The model under review builds one solid part; all positions refer to its coordinate system, in mm. Face numbers are marked on the shaded views. Coordinates: 2 decimals unless noted, no trailing zeros. Write each loop counter-clockwise with the first axis right and the second up, starting at its lowest first coordinate (ties: lowest second). Pieces come first, ordered by that corner, then holes.
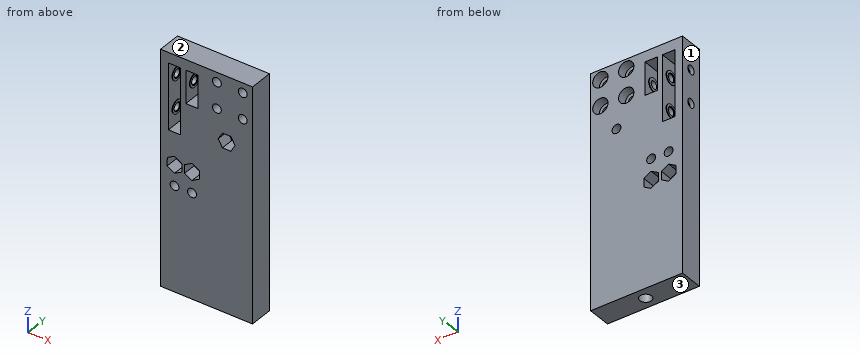
Autodesk Inventor part; units mm, degrees
ref_plane "YZ Plane" through (0, 0, 0) normal (1, 0, 0) x (0, 1, 0)
ref_plane "XZ Plane" through (0, 0, 0) normal (0, 1, 0) x (-1, 0, 0)
ref_plane "XY Plane" through (0, 0, 0) normal (0, 0, 1) x (1, 0, 0)
sketch "Sketch1" plane through (0, 0, 0) normal (0, 1, 0) x (-1, 0, 0)
  line L0 (0, 0) -> (35.5, 0)
  line L1 (35.5, 0) -> (35.5, -90)
  line L2 (35.5, -90) -> (0, -90)
  line L3 (0, -90) -> (0, 0)
  dimension "d0" = 35.5
  dimension "d1" = 90
extrude "Extrusion1" add sketch "Sketch1" along normal blind 9
sketch "Sketch3" plane through (0, 0, 0) normal (0, -1, 0) x (1, 0, 0)
  circle A0 centre (-10, -25) radius 3.25 construction
  line L0 (0, 0) -> (-35.5, 0)
  line L1 (-35.5, 0) -> (-35.5, -90)
  line L2 (-11.6286, -27.8125) -> (-13.25, -24.9958)
  line L3 (-13.25, -24.9958) -> (-11.6214, -22.1833)
  line L4 (-11.6214, -22.1833) -> (-8.3714, -22.1875)
  line L5 (-8.3714, -22.1875) -> (-6.75, -25.0042)
  line L6 (-6.75, -25.0042) -> (-8.3786, -27.8167)
  line L7 (-8.3786, -27.8167) -> (-11.6286, -27.8125)
  line L8 (0, -90) -> (0, 0)
  dimension "d15" = 6.5
  dimension "d16" = 25
  dimension "d26" = 10
extrude "Extrusion3" cut sketch "Sketch3" against normal blind 5
sketch "Sketch5" plane through (0, 9, 0) normal (0, 1, 0) x (1, 0, 0)
  line L0 (0, 0) -> (0, 90)
  line L1 (-35.5, 0) -> (0, 0)
  circle A0 centre (-10, 25) radius 1.7
  dimension "d36" = 3.4
  dimension "d37" = 25
extrude "Extrusion4" cut sketch "Sketch5" against normal through all
sketch "Sketch6" plane through (0, 9, 0) normal (0, 1, 0) x (1, 0, 0)
  line L0 (-32.5, 4) -> (-27.7502, 4)
  line L1 (-27.7502, 4) -> (-27.7502, 29.4)
  line L2 (-27.7502, 29.4) -> (-32.5, 29.4)
  line L3 (-32.5, 29.4) -> (-32.5, 4)
  line L4 (-35.5, 0) -> (0, 0)
  line L5 (-35.5, 90) -> (-35.5, 0)
  line L6 (-25.7502, 4) -> (-21.0002, 4)
  line L7 (-21.0002, 4) -> (-21.0002, 16.7)
  line L8 (-21.0002, 16.7) -> (-25.7502, 16.7)
  line L9 (-25.7502, 16.7) -> (-25.7502, 4)
  line L10 (0, 0) -> (0, 90) construction
  line L11 (-35.5, 90) -> (0, 90)
  line L12 (0, 0) -> (-20, 0) construction
  line L13 (-20, 0) -> (-20, 90) construction
  line L14 (-20, 90) -> (0, 90) construction
  line L15 (0, 90) -> (0, 0)
  circle A0 centre (-23.3752, 41.7) radius 1.7
  circle A1 centre (-30.125, 41.7) radius 1.7
  circle A2 centre (-30.125, 49.7) radius 1.7
  circle A3 centre (-23.3752, 49.7) radius 1.7
  dimension "d43" = 4.7498
  dimension "d44" = 25.4
  dimension "d45" = 4
  dimension "d46" = 3
  dimension "d47" = 4.75
  dimension "d48" = 2
  dimension "d49" = 20
  dimension "d50" = 3.4
  dimension "d90" = 3.4
  dimension "d91" = 5.375
  dimension "d92" = 3.4
  dimension "d93" = 8
  dimension "d94" = 3.4
  dimension "d99" = 40.3
extrude "Extrusion5" cut sketch "Sketch6" against normal through all contours L3 L2 L1 L0 | L9 L8 L7 L6 | A0 | A1 | A2 | A3
sketch "Sketch7" plane through (0, 0, 0) normal (0, -1, 0) x (1, 0, 0)
  circle A0 centre (-23.3752, -41.7) radius 1.7
  circle A1 centre (-23.3752, -41.7) radius 3.25 construction
  line L0 (-23.3752, -38.45) -> (-20.5606, -40.075)
  line L1 (-20.5606, -40.075) -> (-20.5606, -43.325)
  line L2 (-20.5606, -43.325) -> (-23.3752, -44.95)
  line L3 (-23.3752, -44.95) -> (-26.1898, -43.325)
  line L4 (-26.1898, -43.325) -> (-26.1898, -40.075)
  line L5 (-26.1898, -40.075) -> (-23.3752, -38.45)
  line L6 (0, 0) -> (-35.5, 0)
  circle A2 centre (-30.125, -41.7) radius 3.25 construction
  line L7 (-35.5, 0) -> (-35.5, -90)
  line L8 (-30.1645, -44.9498) -> (-32.9591, -43.2907)
  line L9 (-32.9591, -43.2907) -> (-32.9196, -40.0409)
  line L10 (-32.9196, -40.0409) -> (-30.0855, -38.4502)
  line L11 (-30.0855, -38.4502) -> (-27.2909, -40.1093)
  line L12 (-27.2909, -40.1093) -> (-27.3304, -43.3591)
  line L13 (-27.3304, -43.3591) -> (-30.1645, -44.9498)
  dimension "d88" = 6.5
  dimension "d54" = 6.5
  dimension "d87" = 41.7
  dimension "d89" = 5.375
extrude "Extrusion6" cut sketch "Sketch7" against normal blind 5
sketch "Sketch8" plane through (-35.5, 0, -90) normal (-1, 0, 0) x (0, 0, 1)
  circle A0 centre (79.65, 4.5) radius 1.4605
  line L0 (0, 9) -> (90, 9)
  line L1 (90, 0) -> (90, 9)
  circle A1 centre (66.95, 4.5) radius 1.4605
  dimension "d57" = 2.921
  dimension "d58" = 4.5
  dimension "d59" = 10.35
  dimension "d103" = 2.921
  dimension "d104" = 4.5
  dimension "d105" = 12.7
hole "Hole1" at (-35.5, 4.5, -10.35) at (-35.5, 4.5, -23.05) direction (1, 0, 0) diameter 2.921 depth 21 counterbore diameter 3.4 counterbore depth 1.5
sketch "Sketch9" plane through (-21.0002, 9, -16.7) normal (-1, 0, 0) x (0, 0, 1)
  circle A0 centre (6.35, -4.5) radius 1.4605
  circle A1 centre (6.35, -4.5) radius 2.54
  point P0 (16.7, -9)
  dimension "d67" = 5.08
extrude "Extrusion7" add sketch "Sketch9" along normal blind 0.2032
sketch "Sketch10" plane through (-27.7502, 9, -29.4) normal (-1, 0, 0) x (0, 0, 1)
  circle A0 centre (6.35, -4.5) radius 1.7
  circle A1 centre (6.35, -4.5) radius 2.54
  circle A2 centre (19.05, -4.5) radius 2.54
  circle A3 centre (19.05, -4.5) radius 2.54
  circle A4 centre (19.05, -4.5) radius 1.7
  point P0 (29.4, -9)
  dimension "d70" = 5.08
  dimension "d106" = 3.4
extrude "Extrusion8" add sketch "Sketch10" along normal blind 0.2032
sketch "Sketch11" plane through (-25.7502, 9, -4) normal (1, 0, 0) x (0, 0, -1)
  circle A0 centre (6.35, -4.5) radius 1.7
  circle A1 centre (6.35, -4.5) radius 2.54
  point P0 (-4, -9)
  dimension "d73" = 5.08
extrude "Extrusion9" add sketch "Sketch11" along normal blind 0.2032
sketch "Sketch12" plane through (-32.5, 9, -4) normal (1, 0, 0) x (0, 0, -1)
  circle A0 centre (6.35, -4.5) radius 1.7
  circle A1 centre (6.35, -4.5) radius 2.54
  circle A2 centre (19.05, -4.5) radius 1.4605
  circle A3 centre (19.05, -4.5) radius 2.54
  circle A4 centre (19.05, -4.5) radius 1.7
  point P0 (-4, -9)
  dimension "d76" = 5.08
  dimension "d107" = 5.08
  dimension "d108" = 3.4
extrude "Extrusion10" add sketch "Sketch12" along normal blind 0.2032 contours A1 | A3
sketch "Sketch14" plane through (0, 0, -90) normal (0, 0, -1) x (-1, 0, 0)
  circle A0 centre (18, 4.5) radius 2.25
  line L0 (35.5, 0) -> (0, 0)
  line L1 (0, 0) -> (0, 9)
  dimension "d82" = 4.5
  dimension "d83" = 4.5
  dimension "d84" = 18
extrude "Extrusion11" cut sketch "Sketch14" against normal blind 41
sketch "Sketch15" plane through (0, 9, 0) normal (0, 1, 0) x (1, 0, 0)
  circle A0 centre (-30.125, 49.7) radius 1.7
  circle A1 centre (-30.125, 49.7) radius 3.25 construction
  circle A2 centre (-23.3752, 49.7) radius 1.7
  circle A3 centre (-23.3752, 49.7) radius 3.25 construction
  line L0 (-30.125, 52.95) -> (-27.3104, 51.325)
  line L1 (-27.3104, 51.325) -> (-27.3104, 48.075)
  line L2 (-27.3104, 48.075) -> (-30.125, 46.45)
  line L3 (-30.125, 46.45) -> (-32.9396, 48.075)
  line L4 (-32.9396, 48.075) -> (-32.9396, 51.325)
  line L5 (-32.9396, 51.325) -> (-30.125, 52.95)
  line L6 (-23.3752, 52.95) -> (-20.5606, 51.325)
  line L7 (-20.5606, 51.325) -> (-20.5606, 48.075)
  line L8 (-20.5606, 48.075) -> (-23.3752, 46.45)
  line L9 (-23.3752, 46.45) -> (-26.1898, 48.075)
  line L10 (-26.1898, 48.075) -> (-26.1898, 51.325)
  line L11 (-26.1898, 51.325) -> (-23.3752, 52.95)
  point P0 (0, 0)
  dimension "d95" = 6.5
  dimension "d96" = 6.5
extrude "Extrusion12" cut sketch "Sketch15" against normal blind 5
sketch "Sketch17" plane through (0, 9, 0) normal (0, 1, 0) x (1, 0, 0)
  arc A0 (-2.6064, 3.3135) -> (-3.3135, 2.6064) centre (-3.77, 3.77) ccw construction
  arc A1 (-14.2265, 2.6064) -> (-14.9336, 3.3135) centre (-13.77, 3.77) ccw construction
  arc A2 (-14.9336, 14.2265) -> (-14.2265, 14.9336) centre (-13.77, 13.77) ccw construction
  arc A3 (-3.3135, 14.9336) -> (-2.6064, 14.2265) centre (-3.77, 13.77) ccw construction
  point P0 (0, 0)
hole "Hole2" at (-3.77, 9, -3.77) at (-13.77, 9, -3.77) at (-13.77, 9, -13.77) at (-3.77, 9, -13.77) direction (0, -1, 0) diameter 3.4 end through all counterbore diameter 5.9 counterbore depth 3.5
properties part number "Fixed top coupler"
Item 1: To check wall thickness, follow line 1 along Z through (x, y) = (-13.77, 2); line 2 along Z through (x, y) = (-15.5, 4.5); line 3 along Z through (x, y) = (-29.5, 5.5). State the ranges of each line that lie inside material, in increasing order.
Solved:
line 1: z = -90 to -15.47, -12.07 to -5.47, -2.07 to 0
line 2: z = -90 to -24.51, -21.59 to -11.81, -8.89 to 0
line 3: z = -90 to -52.59, -46.81 to -43.28, -40.12 to -29.4, -4 to 0
Item 2: Take a section at B-B, the plane x = -18. Write out the cut boundary in (y, z).
Solved:
outline: (0, -90) - (2.25, -90) - (2.25, -49) - (6.75, -49) - (6.75, -90) - (9, -90) - (9, 0) - (0, 0) - close; hole circle Ø2.92 at (4.5, -23.05); hole circle Ø2.92 at (4.5, -10.35)
Item 3: For pin 1 (1.7 mm diameter, centred on y = 5, z = -23, fed in from -X); pin 2 (4.5 mm diameter, centred on x = -3.77, z = -3.77, fed in from +Y), all flat-tipped, find the tip position at first contact; note any pin that passes through.
Solved:
pin 1: stops at x = -14.5
pin 2: stops at y = 5.5
Item 4: Take a section at A-A, the plane z = -13.77. Write out the cut boundary in (x, y), plus the area to 3 significant figures.
Solved:
outline: (-35.5, 0) - (-32.5, 0) - (-32.5, 9) - (-35.5, 9) - close; (-27.75, 0) - (-25.75, 0) - (-25.75, 9) - (-27.75, 9) - close; (-21, 0) - (-15.47, 0) - (-15.47, 5.5) - (-16.72, 5.5) - (-16.72, 9) - (-21, 9) - close; (-12.07, 0) - (-5.47, 0) - (-5.47, 5.5) - (-6.72, 5.5) - (-6.72, 9) - (-10.82, 9) - (-10.82, 5.5) - (-12.07, 5.5) - close; (-2.07, 0) - (0, 0) - (0, 9) - (-0.82, 9) - (-0.82, 5.5) - (-2.07, 5.5) - close
area: 155 mm2
Item 5: Mouldability with a two-part tool opening along Z and no side actions: class the marked faces 1, 2 and 3 as pulls with the +Z half, pulls with the -Z half, needs draft (parallel to the pull), parting line crosses it, or undercut.
Solved:
face 1: needs draft
face 2: pulls with the +Z half
face 3: pulls with the -Z half
Item 6: Take a section at C-C, the plane x = -10. Write out the cut boundary in (y, z).
Solved:
outline: (0, -90) - (9, -90) - (9, -26.7) - (5, -26.7) - (5, -27.81) - (0, -27.81) - close; (0, -22.19) - (5, -22.19) - (5, -23.3) - (9, -23.3) - (9, 0) - (0, 0) - close
Item 7: Take a section at D-D, the plane z = -64.5. Write out the cut boundary in (x, y), plus the area to 3 significant figures.
Solved:
outline: (-35.5, 0) - (0, 0) - (0, 9) - (-35.5, 9) - close; hole circle Ø4.5 at (-18, 4.5)
area: 304 mm2
